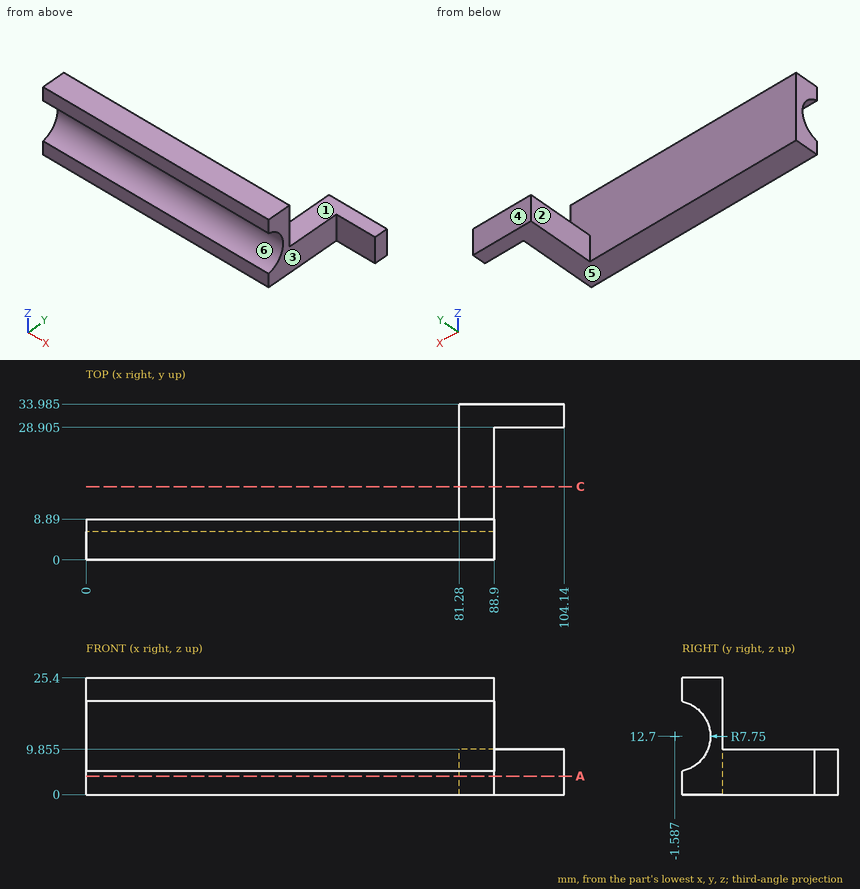
Geometry check sheet. Reference: drawing and pictorial views, mm from the part's lowest x, y, z. A direction names the side the tool comes from. Coordinates: 2 decimals unless noted, no trailing zeros. Write each loop counter-clockwise with the first axis right and the second up, starting at its lowest first coordinate (ties: lowest second). Pieces come first, ordered by that corner, then holes. Notation, with made-up numbers: (-23.5, -23) - (23.5, -23) arc R24 ccw to (23.5, 7) - close; hole circle Ø11 at (-12.5, 42). An arc over 180 degrees is marked (long way). One line per question, with ' | ' between items. Start each with the question number.
1. Section check A-A (z = 4). Enter the section's corners in (x, y) (1 decimal), plus the area to 3 significant figures.
2. Access from +Z, -Z, +X, -X, +Y, -Y to the whole of each face (thin tool, end or side, straight path). Record for the marked faces 1, 2 and 3.
3. Section check C-C (y = 16). Enter the section's corners in (x, z) (1 decimal), plus the area to 3 significant figures.
4. Material ranges on line 1 along Y through (x, z) = (62, 20.5); line 2 along Y through (x, z) = (77, 12.25); line 3 along X through (y, z) = (12, 8), recorded low to high.
5. Draft check along Z on the marked faces 4, 5 and 6. Enter one of: released by +Z, released by -Z, zero draft, split by the parting line, or undercut.
6. Gauge pin test, flat ends, axial feed: P1, Ø1, axis at x = 62.5, z = 15, coming from the +Y side; P2, Ø3, axis at y = 18, z = 3, coming from the -X side; P3, Ø3, axis at x = 89, y = 29, coming from the +Z side (1 decimal). Record the tip position at first contact, or that the pin passes through.
Computed values:
1) outline: (0, 0) - (88.9, 0) - (88.9, 28.9) - (104.1, 28.9) - (104.1, 34) - (81.3, 34) - (81.3, 8.9) - (0, 8.9) - close | area: 1,060 mm²
2) face 1: +Z, +X, -X, +Y | face 2: +Z, -Z, -X, +Y | face 3: +Z, -Z, +X, -Y
3) outline: (81.3, 0) - (88.9, 0) - (88.9, 9.9) - (81.3, 9.9) - close | area: 75.1 mm²
4) line 1: 0 to 8.89 | line 2: 6.15 to 8.89 | line 3: 81.28 to 88.9
5) face 4: zero draft | face 5: released by -Z | face 6: undercut
6) P1: y = 8.89 | P2: x = 81.28 | P3: z = 9.9
